Geometry check sheet. Reference: the model listing, model coordinates, mm. A direction names the side the tool comes from. Round coordinates to 2 decimals unless told otherwise and drop trailing zeros. Loops run counter-clockwise (first coordinate to the right, second up) from the corner with the lowest first, then second, coordinate; pieces in that order, holes last. Notation, with made-up numbers: M -32,24.25 L -26,24.25 A22 cw -26,39.25 Z; hole C 44.5,67 d3. An arc over 180 degrees is marked long. Write item = value, one per line.
Autodesk Inventor part; units mm, degrees
ref_plane "YZ Plane" through (0, 0, 0) normal (1, 0, 0) x (0, 1, 0)
ref_plane "XZ Plane" through (0, 0, 0) normal (0, 1, 0) x (-1, 0, 0)
ref_plane "XY Plane" through (0, 0, 0) normal (0, 0, 1) x (1, 0, 0)
sketch "Sketch1" plane through (0, 0, 0) normal (0, 1, 0) x (-1, 0, 0)
  line L0 (0, 0) -> (9.5, 0)
  line L1 (9.5, 0) -> (9.5, -64)
  line L2 (9.5, -64) -> (0, -64)
  line L3 (0, -64) -> (0, 0)
  circle A0 centre (3.7, -11.5) radius 2.25
  circle A1 centre (3.7, -59.5) radius 2.25
  line L4 (3.7, -11.5) -> (3.7, -59.5) construction
  dimension "d1" = 9.5
  dimension "d2" = 64
  dimension "d3" = 4.5
  dimension "d4" = 48
  dimension "d6" = 3.7
  dimension "d17" = 4.5
extrude "Extrusion1" add sketch "Sketch1" along normal blind 12
sketch "Sketch2" plane through (-9.5, 0, 0) normal (0, 0, 1) x (1, 0, 0)
  line L0 (9.5, 12) -> (0, 12)
  line L1 (3, 12) -> (8.4, 12)
  line L2 (8.4, 12) -> (8.4, 10.8)
  line L3 (8.4, 10.8) -> (3, 10.8)
  line L4 (3, 10.8) -> (3, 12)
  line L5 (9.5, 0) -> (9.5, 12)
  line L6 (3.55, 0) -> (8.05, 0)
  line L7 (3.55, 12) -> (8.05, 12)
  line L8 (9.5, 0) -> (9.5, 12)
  line L9 (9.5, 0) -> (9.5, 12)
  line L10 (3.55, 12) -> (8.05, 12)
  line L11 (3.55, 12) -> (3.55, 0)
  line L12 (3.55, 12) -> (8.05, 12)
  line L13 (3.55, 0) -> (8.05, 0)
  line L14 (3.55, 12) -> (8.05, 12)
  line L15 (3.55, 0) -> (8.05, 0)
  line L16 (3.55, 12) -> (8.05, 12)
  line L17 (3.55, 0) -> (8.05, 0)
  dimension "d9" = 1.1
  dimension "d10" = 5.4
  dimension "d11" = 1.2
  dimension "d76" = 12
extrude "Extrusion2" cut sketch "Sketch2" against normal up to next
sketch "Sketch3" plane through (0, 0, 0) normal (0, -1, 0) x (1, 0, 0)
  circle A0 centre (-3.7, -11.5) radius 2.25
  circle A1 centre (-3.7, -11.5) radius 3.75
  circle A2 centre (-3.7, -59.5) radius 2.25
  circle A3 centre (-3.7, -59.5) radius 3.75
  point P0 (0, 0)
  dimension "d14" = 7.5
extrude "Extrusion3" cut sketch "Sketch3" against normal blind 3
fillet "Fillet1" radius 1 4 edges at (0, 1.5, -58.8897) (0, 1.5, -60.1103) (0, 1.5, -10.8897) (0, 1.5, -12.1103)
fillet "Fillet2" radius 4 2 edges at (-9.5, 6, -64) (-9.5, 6, 0)
sketch "Sketch28" plane through (0, 0, 0) normal (0, -1, 0) x (1, 0, 0)
  arc A0 (-1.5684, -56.4147) -> (0, -55.592) centre (-1, -55.592) ccw
  line L0 (0, -55.592) -> (0, -53)
  line L1 (0, -15.408) -> (0, -55.592)
  line L2 (-9.5, -60) -> (-9.5, -4)
  line L3 (0, -53) -> (-9.5, -53)
  line L4 (-9.5, -53) -> (-9.5, -34)
  line L5 (-9.5, -34) -> (0, -34)
  line L6 (0, -34) -> (0, -53)
  point P0 (0, 0)
  point P1 (0, -34)
  dimension "d107" = 2.592
  dimension "d108" = 19
extrude "Extrusion19" add sketch "Sketch28" along normal blind 20
sketch "Sketch40" plane through (0, -20, 0) normal (0, -1, 0) x (1, 0, 0)
  line L0 (0, -53) -> (-9.5, -53)
  line L1 (-9.5, -53) -> (-9.5, -73)
  line L2 (-9.5, -73) -> (0, -73)
  line L3 (0, -73) -> (0, -43)
  line L4 (0, 0) -> (0, -64)
  line L5 (0, -43) -> (-9.5, -43)
  line L6 (-9.5, -43) -> (-9.5, -53)
  line L7 (-9.5, -43) -> (0, -43)
  line L8 (0, -43) -> (0, -73)
  line L9 (0, -73) -> (-9.5, -73)
  line L10 (-9.5, -73) -> (-9.5, -43)
  dimension "d130" = 20
  dimension "d131" = 30
extrude "Extrusion21" add sketch "Sketch40" along normal blind 10
sketch "Sketch41" plane through (0, 0, -53) normal (0, 0, -1) x (-1, 0, 0)
  point P0 (0, 0)
sketch "Sketch42" plane through (0, -30, 0) normal (0, -1, 0) x (1, 0, 0)
  line L0 (-9.5, -73) -> (0, -73)
  line L1 (-9.5, -73) -> (-40.7, -73)
  line L2 (-9.5, -73) -> (21.7, -73) construction
  line L3 (-40.7, -73) -> (-40.7, -66)
  line L4 (-40.7, -66) -> (9.3, -66)
  line L5 (9.3, -66) -> (9.3, -73)
  line L6 (9.3, -73) -> (-9.5, -73)
  point P0 (0, 0)
  point P1 (0, -73)
  dimension "d134" = 31.2
  dimension "d135" = 180
  dimension "d136" = 7
  dimension "d137" = 50
  dimension "d138" = 7
extrude "Extrusion22" add sketch "Sketch42" along normal blind 7
sketch "Sketch43" plane through (-40.7, -30, -73) normal (-1, 0, 0) x (0, 0, 1)
  arc A0 (7, -7) -> (7, -57) centre (31.4949, -32) ccw
  point P0 (73, 30)
  dimension "d141" = 50
  dimension "d142" = 35
sketch "Sketch44" plane through (0, -37, 0) normal (0, -1, 0) x (1, 0, 0)
  line L0 (9.3, -73) -> (9.3, -66)
  line L1 (-40.7, -73) -> (-9.5, -73)
  line L2 (9.3, -66) -> (-40.7, -66)
  line L3 (-40.7, -66) -> (-40.7, -73)
  line L4 (-40.7, -73) -> (9.3, -73)
  line L5 (9.3, -73) -> (9.3, -66)
  point P0 (0, 0)
  point P1 (-9.5, -73)
sweep "Sweep3" add profiles "Sketch44" path "Sketch43"
sketch "Sketch46" plane through (-40.7, -30, -73) normal (-1, 0, 0) x (0, 0, 1)
  arc A0 (7, -7) -> (7, -57) centre (31.4949, -32) ccw
  circle A1 centre (31.4949, -32) radius 35 construction
  line L0 (31.4949, -32) -> (3.353, -60.7222)
  arc A2 (0, -7) -> (7.1429, -63.9985) centre (31.4949, -32) ccw
  line L1 (31.4949, -32) -> (7.1429, -63.9985)
  point P0 (73, 30)
extrude "Extrusion23" cut sketch "Sketch46" against normal up to surface (50 mm away)
sketch "Sketch47" plane through (-40.7, -87, -66) normal (0, -0.6998542, 0.7142857) x (1, 0, 0)
  line L0 (0, 30.8153) -> (0, -5.2111)
  line L1 (0, -3.2111) -> (50, -3.2111) construction
  line L2 (50, 30.8153) -> (50, -5.2111)
  line L3 (50, 0) -> (0, 0)
  line L4 (0, 0) -> (25, -6.4221) construction
  line L5 (25, -6.4221) -> (50, 0) construction
  spline S0 degree 2 poles (0, 0) (25, -6.4221) (50, 0) knots 1 1 1 2 2 2
  line L6 (0, 0) -> (50, 0)
  line L7 (50, -5.2111) -> (0, -5.2111)
  line L8 (60.7, 35) -> (-10.7, 35)
  point P0 (40.7, 108.3332)
  dimension "d149" = 2
revolve "Revolution2" cut sketch "Sketch47" angle 90 about axis through (-15.7, -62, -41.5051) along (1, 0, 0) contours L3 S0
sketch "Sketch48" plane through (-40.7, -90.7222, -69.647) normal (0, -0.6998542, 0.7142857) x (1, 0, 0)
  point P0 (40.7, 113.5443)
properties part number "Back"
(1) Material ranges on line 1 along Z through (x, y) = (-3.7, 4.75); line 2 along Z through (x, y) = (-3.7, 1.75); line 3 along X through (y, z) = (5.5, -11.5), recorded low to high. Write a range as from..to.
Result set:
line_1 = -64..-61.75, -57.25..-13.75, -9.25..0
line_2 = -64..-63.25, -55.75..-15.25, -7.75..0
line_3 = -9.5..-5.95, -1.45..0
(2) Depth check by flat-ended pin: pin 1 Ø10 at (x, z) = (-3.7, -11.5) entering from -Y; pin 2 Ø10 at (y, z) = (-29.5, -49.5) entering from -X; pin 3 Ø10 at (x, z) = (1.5, -65) entering from -Y; pin 4 Ø5 at (x, z) = (-5.5, -60) entering from +Y. Enter the tip coordinate at first touch or a pass-through.
Result set:
pin_1 = 0
pin_2 = -9.5
pin_3 = -90.72
pin_4 = 12
(3) Tool access check on faces 1 (the flat face through (-5, 0, -17)), 2 (the flat face through (-1, 3, -11)), 3 (the flat face through (-25, -30, -69)). Record the directions out of +Z, -Z, +X, -X, +Y, -Y that give a thin tool (end or side, any length) a straight path to the whole face; none if there is none.
Result set:
face_1 = +Z, +X, -X, -Y
face_2 = -Y
face_3 = +Z, -Z, -X, +Y
(4) Sectioned sample at A-A on z = -11.5. Record the cut outline in (x, y), then the cut area to 3 significant figures.
Result set:
outline = M -9.5,0 L -7.45,0 L -7.45,3 L -5.95,3 L -5.95,10.8 L -6.5,10.8 L -6.5,12 L -9.5,12 Z; M -1.45,3 L 0,3 L 0,12 L -1.1,12 L -1.1,10.8 L -1.45,10.8 Z
area = 50.1 mm2
(5) Sectioned sample at C-C on y = -18.5. Record the cut outline in (x, z), then the cut area to 4 significant figures.
Result set:
outline = M -9.5,-53 L 0,-53 L 0,-34 L -9.5,-34 Z
area = 180.5 mm2
(6) Release check for a two-part mould opening along Z. For faces 4 (the flat face through (-1, 3, -59)), 5 (the flat face through (-5, -10, -34)), 6 (the flat face through (-15, -32, -73)) record: released by +Z, released by -Z, zero draft, split by the parting line, or undercut.
Result set:
face_4 = undercut
face_5 = released by +Z
face_6 = released by -Z
(7) Sectioned sample at B-B on z = -41. Record the cut outline in (x, y), then the cut area to 3 significant figures.
Result set:
outline = M -9.5,-20 L 0,-20 L 0,12 L -1.1,12 L -1.1,10.8 L -6.5,10.8 L -6.5,12 L -9.5,12 Z
area = 298 mm2
(8) Sectioned sample at D-D on x = -3.7. State how many separate pieces and enclosed holes the cut face has, then the cut area to 3 significant figures.
Result set:
separate_pieces = 3
enclosed_holes = 0
area = 1,460 mm2
